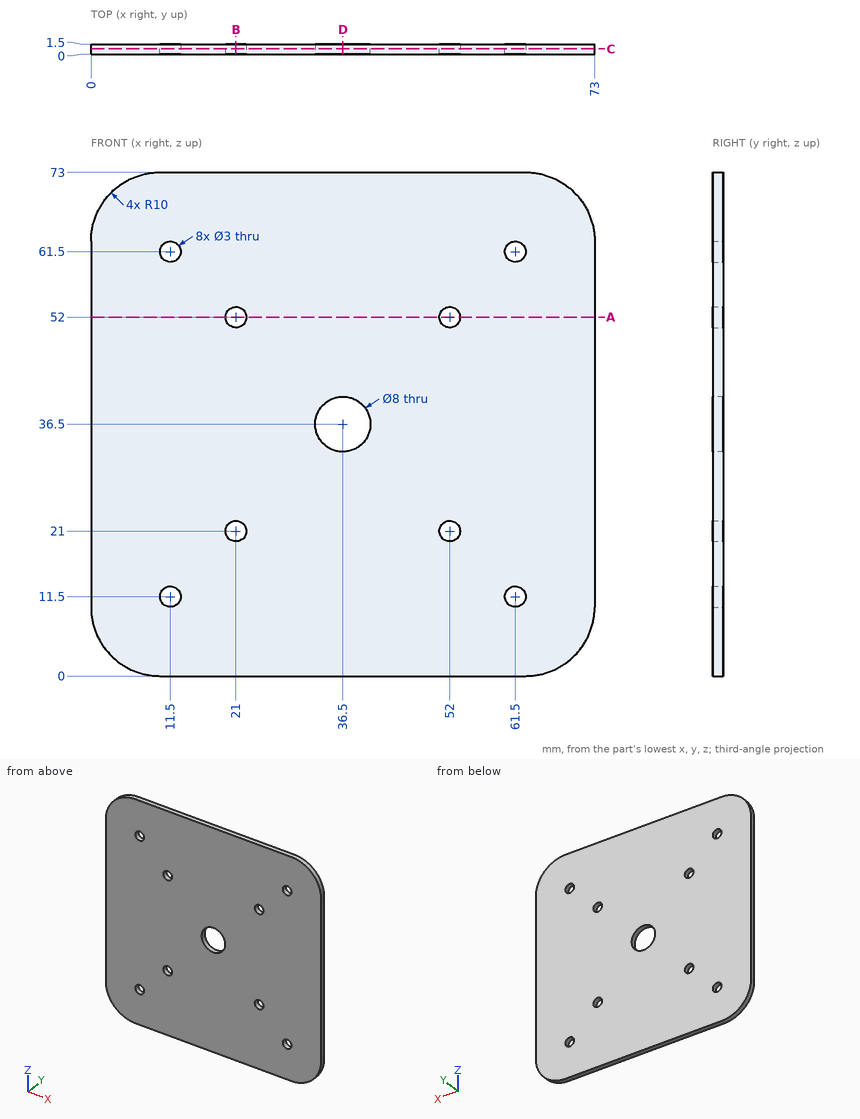
Here's the drawing with two shaded views (mm, measured from the low corner). I have some questions. Give positions to 0.01 mm unless a question says otherwise; leave off trailing zeros. Write each loop counter-clockwise with the first axis right and the second up, starting at its lowest first coordinate (ties: lowest second). Pieces come first, ordered by that corner, then holes. Notation, with made-up numbers: (-31.5, 8) -> (19.5, 8) arc R22 ccw to (19.5, 44) -> close; hole circle Ø3 at (-2.75, 37). An arc over 180 degrees is marked (long way). One line per item, written item: value.
Q1. Imagine slicing it at D-D on x = 36.5. Please give me the cut outline in (y, z).
Results found:
outline: (0, 0) -> (1.5, 0) -> (1.5, 32.5) -> (0, 32.5) -> close; (0, 40.5) -> (1.5, 40.5) -> (1.5, 73) -> (0, 73) -> close
Q2. For P1, Ø1.8, axis at x = 52, z = 52, coming from the -Y side; P2, Ø3.5, axis at x = 52, z = 21, coming from the -Y side, each with a flat end and sliding along its axis, tell me the tip position at first contact or that it passes through.
Results found:
P1: passes through
P2: stops at y = 0
Q3. Imagine slicing it at C-C on y = 0.8. Give the number of separate pieces and of enclosed holes in the cut face, and give its area (3 significant figures).
Results found:
separate pieces: 1
enclosed holes: 9
area: 5,140 mm^2
Q4. Please list where these lines run through material, in increasing order: line 1 (X direction, y = 0.5, z = 61.5); line 2 (X direction, y = 0.5, z = 21). Write a range as [from, to].
Results found:
line 1: x = [0, 10], [13, 60], [63, 73]
line 2: x = [0, 19.5], [22.5, 50.5], [53.5, 73]
Q5. Imagine slicing it at A-A on z = 52. Please give me the cut outline in (x, y), and give its area (4 significant figures).
Results found:
outline: (0, 0) -> (19.5, 0) -> (19.5, 1.5) -> (0, 1.5) -> close; (22.5, 0) -> (50.5, 0) -> (50.5, 1.5) -> (22.5, 1.5) -> close; (53.5, 0) -> (73, 0) -> (73, 1.5) -> (53.5, 1.5) -> close
area: 100.5 mm^2
Q6. Imagine slicing it at B-B on x = 21. Please give me the cut outline in (y, z), and give its area (4 significant figures).
Results found:
outline: (0, 0) -> (1.5, 0) -> (1.5, 19.5) -> (0, 19.5) -> close; (0, 22.5) -> (1.5, 22.5) -> (1.5, 50.5) -> (0, 50.5) -> close; (0, 53.5) -> (1.5, 53.5) -> (1.5, 73) -> (0, 73) -> close
area: 100.5 mm^2
